The listing builds one solid part. Answer for the finished solid, in the listing's coordinates (mm). Coordinates: 2 decimals unless noted, no trailing zeros. Write each loop counter-clockwise with the first axis right and the second up, starting at its lowest first coordinate (ties: lowest second). Pieces come first, ordered by that corner, then holes.
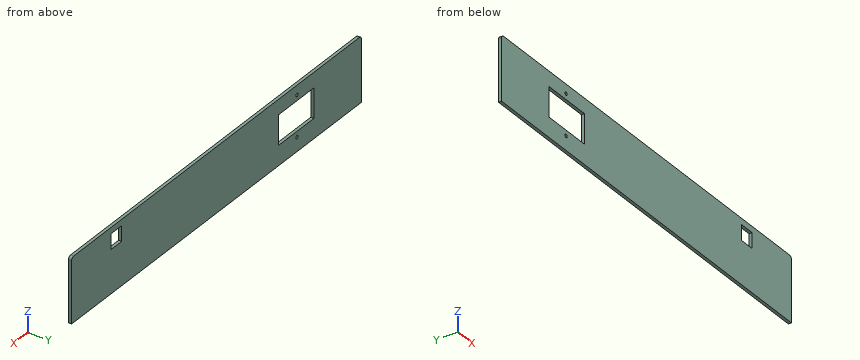
from build123d import *

# Parameters (mm, degrees)
F0_R     = 1.6
F0_W     = 50
F0_H     = 29
F0_W_2   = 15
F0_H_2   = 15
F1_DEPTH = 3


with BuildPart() as f1:
    # F0 (on Front) → F1 (new body)
    with BuildSketch(Plane.XZ):
        with BuildLine():
            Line((176.212173, -52.694491), (-225.787827, -52.694491))
            ThreePointArc((-225.787827, -52.694491), (-227.909148, -53.57317), (-228.787827, -55.694491))
            Line((-228.787827, -55.694491), (-228.787827, -115.694491))
            Line((-228.787827, -115.694491), (179.212173, -115.694491))
            Line((179.212173, -115.694491), (179.212173, -55.694491))
            ThreePointArc((179.212173, -55.694491), (178.333493, -53.57317), (176.212173, -52.694491))
        make_face()
        with Locations((-137.990355, -101.892883)):
            Circle(F0_R, mode=Mode.SUBTRACT)
        with Locations((-136.990355, -81.892883)):
            Rectangle(F0_W, F0_H, mode=Mode.SUBTRACT)
        with Locations((-137.990355, -61.892883)):
            Circle(F0_R, mode=Mode.SUBTRACT)
        with Locations((116.212173, -66.194491)):
            Rectangle(F0_W_2, F0_H_2, mode=Mode.SUBTRACT)
    extrude(amount=F1_DEPTH)


solid = f1.part
Q1. The part is cut by section A-A, the plane z = -82.5. Write down the section's boundary in (x, y).
Answers below:
outline: (-228.79, -3) - (-161.99, -3) - (-161.99, 0) - (-228.79, 0) - close; (-111.99, -3) - (179.21, -3) - (179.21, 0) - (-111.99, 0) - close
Q2. Given pin 1 (5 mm diameter, centred on x = -137.99, z = -101.89, fed in from -Y), flat-ended and moving along its own axis, determine where the tip first touches the part or whether it passes through.
Answers below:
pin 1: stops at y = -3
Q3. The part is cut by section B-B, the plane y = -1.5. Write down the section's boundary in (x, z), then the cut area to 3 significant figures.
Answers below:
outline: (-228.79, -115.69) - (179.21, -115.69) - (179.21, -55.69) arc R3 ccw to (176.21, -52.69) - (-225.79, -52.69) arc R3 ccw to (-228.79, -55.69) - close; hole (-161.99, -96.39) - (-111.99, -96.39) - (-111.99, -67.39) - (-161.99, -67.39) - close; hole circle Ø3.2 at (-137.99, -101.89); hole circle Ø3.2 at (-137.99, -61.89); hole (108.71, -73.69) - (123.71, -73.69) - (123.71, -58.69) - (108.71, -58.69) - close
area: 24,000 mm2
Q4. Find the intervals of material crossed by probe 1 along X at (y, z) = (-0.75, -70.5); probe 2 along X at (y, z) = (-2.7, -96); probe 3 along X at (y, z) = (-1.05, -102), in increasing order.
Answers below:
probe 1: x = -228.79 to -161.99, -111.99 to 108.71, 123.71 to 179.21
probe 2: x = -228.79 to -161.99, -111.99 to 179.21
probe 3: x = -228.79 to -139.59, -136.39 to 179.21
